```python
from build123d import *

# Parameters (mm, degrees)
SKETCH_1_W          = 24
SKETCH_1_H          = 6
EXTRUDE_1_DEPTH     = 16
CUT_EXTRUDE_1_DEPTH = 13
CUT_EXTRUDE_START   = -11.7
CUT_EXTRUDE_6_DEPTH = 1.3


with BuildPart() as part:
    # Эскиз1 → Бобышка-Вытянуть1 (new body)
    with BuildSketch(Plane(origin=(0, 0, 0), x_dir=(0, 0, -1), z_dir=(1, 0, 0))):
        with Locations((12, 3)):
            Rectangle(SKETCH_1_W, SKETCH_1_H)
    extrude(amount=EXTRUDE_1_DEPTH)

    # Эскиз2 → Вырез-Вытянуть1 (cut)
    with BuildSketch(Plane(origin=(16, 0, 0), x_dir=(0, 0, -1), z_dir=(1, 0, 0))):
        with BuildLine():
            ThreePointArc((16.800735254, 0), (10, 2.5), (3.199264746, 0))
            Line((3.199264746, 0), (16.800735254, 0))
        make_face()
    extrude(amount=-CUT_EXTRUDE_1_DEPTH, mode=Mode.SUBTRACT)

    # Эскиз3 → Вырез-Вытянуть6 (cut)
    with BuildSketch(Plane(origin=(16, 0, 0), x_dir=(0, 0, -1), z_dir=(1, 0, 0)).offset(CUT_EXTRUDE_START)):
        with BuildLine():
            Line((11.871529868, 2.331862173), (4.350732789, 6))
            Line((4.350732789, 6), (0, 6))
            Line((0, 6), (0, 0))
            Line((0, 0), (3.199264746, 0))
            ThreePointArc((3.199264746, 0), (7.273525769, 2.139839164), (11.871529868, 2.331862173))
        make_face()
    extrude(amount=-CUT_EXTRUDE_6_DEPTH, mode=Mode.SUBTRACT)


solid = part.part
```
Model file for the job. Use its own axes, mm. A direction names the side the tool comes from. Coordinates: 2 decimals unless noted, no trailing zeros. Order: outer loops, then holes, each group sorted by start corner. A loop starts at its lowest first (then second) coordinate and runs counter-clockwise, first axis right, second up. Notation, with made-up numbers: M -11.5,-5.75 L 6.5,-5.75 A8 ccw 6.5,6.25 Z; hole C -29,-11 d1. An arc over 180 degrees is marked long. Answer as CSV lines item,"result".
(1) Band-saw the part on D-D, the plane z = -14. List the corners of the cut face in (x, y), then the cut area to 3 significant figures.
Geometry says:
outline,"M 0,0 L 3,0 L 3,1.71 L 16,1.71 L 16,6 L 0,6 Z"
area,"73.8 mm2"
(2) Band-saw the part on C-C, the plane x = 8.75. List the corners of the cut face in (y, z), then the cut area to 3 significant figures.
Geometry says:
outline,"M 0,-24 L 6,-24 L 6,0 L 0,0 L 0,-3.2 A10.5 cw 0,-16.8 Z"
area,"121 mm2"
(3) Pull direction X, two halves, no side cores. Call faces 1 (the flat face through (8, 3, -24)), 2 (the flat face through (3, 2, -6)), 3 (the flat face through (16, 4, -12)): +X half, -X half, draft (parallel to the pull), parting line (faces both ways), or undercut.
Geometry says:
face 1,"draft"
face 2,"undercut"
face 3,"+X half"
(4) Band-saw the part on B-B, the plane y = 4.3. List the corners of the cut face in (x, z), then the cut area to 3 significant figures.
Geometry says:
outline,"M 0,-24 L 16,-24 L 16,0 L 4.3,0 L 4.3,-7.84 L 3,-7.84 L 3,0 L 0,0 Z"
area,"374 mm2"
(5) Wall check: line 1 along X through (y, z) = (4, -5.25); line 2 along X through (y, z) = (0.95, -6.5); line 3 along Z through (x, y) = (11.5, 0.8). Give the ranges that are in metal, low to high.
Geometry says:
line 1,"x = 0 to 3, 4.3 to 16"
line 2,"x = 0 to 3"
line 3,"z = -24 to -15.73, -4.27 to 0"
(6) Flat gauge pins, fed straight in: pin 1 (3 mm diameter, centred on y = 3.5, z = -7.5, fed in from -X); pin 2 (2 mm diameter, centred on x = 6.5, z = -4.5, fed in from -Y). Where does each tip first touch, or does it go through?
Geometry says:
pin 1,"stops at x = 0"
pin 2,"stops at y = 0.25"
(7) Band-saw the part on A-A, the plane z = -2.5. List the corners of the cut face in (x, y), then the cut area to 3 significant figures.
Geometry says:
outline,"M 0,0 L 3,0 L 3,6 L 0,6 Z; M 4.3,0 L 16,0 L 16,6 L 4.3,6 Z"
area,"88.2 mm2"
(8) 3-axis set-ups, long thin cutter, end or side, ignore diameter. For faces 4 (the flat face through (8, 6, -12)), 5 (the cylindrical face through (9.6, 2.5, -10.1)), 6 (the flat face through (4.3, 3, -3)): which of +Z, -Z, +X, -X, +Y, -Y reach the whole face in a straight line?
Geometry says:
face 4,"+Z, -Z, +X, -X, +Y"
face 5,"+X, -Y"
face 6,"+Z, -Y"
